Input: part model. Units: mm. Frame: model coordinates. Round coordinates to 2 decimals unless told otherwise and drop trailing zeros. Loops run counter-clockwise (first coordinate to the right, second up) from the corner with the lowest first, then second, coordinate; pieces in that order, holes last. Notation, with made-up numbers: (87, 8.5) -> (127, 8.5) arc R27 ccw to (127, 30.5) -> close; hole circle Ø7 at (-18.5, 86). An arc over 180 degrees is marked (long way). Answer in a Markdown table with one row per item. Add a question column.
Q1. Mould query, pull axis X, two halves, no side actions, for faces 1 (the face through (0, 0, 3)), 2 (the face through (2.6, 0.4, -1.5)), 3 (the face through (-1.873, -0.416, -0.082)). Classes: pulls with the +X half, pulls with the -X half, needs draft (parallel to the pull), parting line crosses it, or undercut.
Q2. Section A-A, the plane x = 0. Output: boundary loops of the cut face in (y, z) (3 decimals).
Q3. Section B-B, the plane y = -9.5. Output: boundary loops of the cut face in (x, z) (3 decimals).
Q4. Ray query, L1, parallel to X at y = 19.5, z = 1; L2, parallel to X at y = -11.5, z = 0 (3 decimals); L3, parallel to Z at x = 0, y = -11 (3 decimals). Return the intervals inside material, ascending. Write a range as from..to.
Q5. Pin query (flat end, axial travel): pin 1 (2 mm diameter, centred on y = 19.5, z = 2, fed in from +X); pin 2 (1.5 mm diameter, centred on y = -4.5, z = -2, fed in from +X). Return the tip coordinate at first contact, or that it passes through.
```python
from build123d import *

# Parameters (mm, degrees)
SKETCH1_R           = 1.875
BOSS_EXTRUDE1_DEPTH = 30
FILLET1_R           = 0.25


with BuildPart() as part:
    # Sketch1 → Boss-Extrude1 (new body, symmetric)
    with BuildSketch(Plane(origin=(0, 0, 0), x_dir=(1, 0, 0), z_dir=(0, 1, 0))):
        Polygon((1.732050808, 3), (-1.732050808, 3), (-3.464101615, 0), (-1.732050808, -3), (1.732050808, -3), (3.464101615, 0), align=None)
        Circle(SKETCH1_R, mode=Mode.SUBTRACT)
    extrude(amount=BOSS_EXTRUDE1_DEPTH, both=True)

    # Fillet1
    fillet1_edges = [part.edges().sort_by_distance(p)[0] for p in [
        (-2.598076211, 30, -1.5),
        (3.464101615, 0, 0),
        (1.732050808, 0, 3),
        (-1.732050808, 0, 3),
        (-3.464101615, 0, 0),
        (-1.732050808, 0, -3),
        (1.732050808, 0, -3),
        (-2.598076211, 30, 1.5),
        (0, 30, 3),
        (-1.875, -30, 0),
        (-1.875, 30, 0),
        (2.598076211, 30, 1.5),
        (2.598076211, 30, -1.5),
        (2.598076211, -30, 1.5),
        (0, -30, 3),
        (-2.598076211, -30, 1.5),
        (0, 30, -3),
        (-2.598076211, -30, -1.5),
        (0, -30, -3),
        (2.598076211, -30, -1.5),
    ]]
    fillet(fillet1_edges, radius=FILLET1_R)


solid = part.part
```
Answer block:
| question | item | result |
|---|---|---|
| 1 | face 1 | needs draft |
| 1 | face 2 | pulls with the +X half |
| 1 | face 3 | undercut |
| 2 | outline | (-30, -2.75) arc R0.25 ccw to (-29.75, -3) -> (29.75, -3) arc R0.25 ccw to (30, -2.75) -> (30, -2.125) arc R0.25 ccw to (29.75, -1.875) -> (-29.75, -1.875) arc R0.25 ccw to (-30, -2.125) -> close; (-30, 2.125) arc R0.25 ccw to (-29.75, 1.875) -> (29.75, 1.875) arc R0.25 ccw to (30, 2.125) -> (30, 2.75) arc R0.25 ccw to (29.75, 3) -> (-29.75, 3) arc R0.25 ccw to (-30, 2.75) -> close |
| 3 | outline | (-3.392, -0.125) -> (-1.804, -2.875) arc R0.25 ccw to (-1.588, -3) -> (1.588, -3) arc R0.25 ccw to (1.804, -2.875) -> (3.392, -0.125) arc R0.25 ccw to (3.392, 0.125) -> (1.804, 2.875) arc R0.25 ccw to (1.588, 3) -> (-1.588, 3) arc R0.25 ccw to (-1.804, 2.875) -> (-3.392, 0.125) arc R0.25 ccw to start; hole circle Ø3.75 at (0, 0) |
| 4 | L1 | -2.89..-1.59, 1.59..2.89 |
| 4 | L2 | -3.425..-1.875, 1.875..3.425 |
| 4 | L3 | -3..-1.875, 1.875..3 |
| 5 | pin 1 | x = 2.89 |
| 5 | pin 2 | x = 2.74 |
